Verification items for the finished model (mm, model axes). Coordinates: 2 decimals unless noted, no trailing zeros. Order: outer loops, then holes, each group sorted by start corner. A loop starts at its lowest first (then second) coordinate and runs counter-clockwise, first axis right, second up. Notation, with made-up numbers: M 59.5,38 L 83.5,38 A6 cw 83.5,47 Z; hole C 14.25,14 d2. An arc over 180 degrees is marked long. Return JSON: item names as keys, results as strings. Group by question number.
1. Section check A-A, the plane z = -25. Record the cut outline in (x, y), plus the area to 3 significant figures.
2. Section check D-D, the plane x = -93. Record the cut outline in (y, z), plus the area to 3 significant figures.
3. Material ranges on line 1 along X through (y, z) = (0.95, -31.5); line 2 along X through (y, z) = (1.9, -42.5); line 3 along Z through (x, y) = (11, 2.35), recorded low to high.
4. Mould release check, pull along X, two halves, no side actions. Record for faces 1 (the flat face through (103.7, 1.5, -24.9)), 2 (the flat face through (2, 3, 1)), 3 (the cylindrical face through (106.22, 1.48, -70.07)): +X half, -X half, draft (parallel to the pull), parting line (faces both ways), or undercut.
5. Gauge pin test, flat ends, axial feed: pin 1 (0.9 mm diameter, centred on x = 1, y = 1.5, fed in from +Z); pin 2 (1.5 mm diameter, centred on y = 1, z = -13, fed in from -X); pin 3 (1 mm diameter, centred on y = 0.5, z = 9.5, fed in from -X). Record the tip position at first contact, or that the pin passes through.
6. Section check C-C, the plane z = -43. Record the cut outline in (x, y).
7. Section check B-B, the plane y = 2.35. Give the number of separate pieces and of enclosed holes in the cut face, plus the area to 3 significant figures.
```python
from build123d import *

# Parameters (mm, degrees)
EXTRUDE_1_DEPTH     = 3
CUT_EXTRUDE_START   = -10
CUT_EXTRUDE_1_DEPTH = 10
SKETCH_3_R          = 1.75
CUT_EXTRUDE_2_DEPTH = 10
CUT_EXTRUDE_3_DEPTH = 10


with BuildPart() as part:
    # 草图1 → 凸台-拉伸1 (new body)
    with BuildSketch(Plane(origin=(0, 0, 0), x_dir=(1, 0, 0), z_dir=(0, 1, 0))):
        with BuildLine():
            Line((-66.78059141, 154.593992167), (66.78059141, 154.593992167))
            ThreePointArc((66.78059141, 154.593992167), (85.265515034, 148.222525736), (95.898700635, 131.814498742))
            Line((95.898700635, 131.814498742), (111.265547961, 69.844672358))
            ThreePointArc((111.265547961, 69.844672358), (112.147438737, 62.624165782), (111.265547961, 55.403659207))
            Line((111.265547961, 55.403659207), (95.898700635, -6.566167178))
            ThreePointArc((95.898700635, -6.566167178), (85.265515034, -22.974194171), (66.78059141, -29.345660602))
            Line((66.78059141, -29.345660602), (-66.78059141, -29.345660602))
            ThreePointArc((-66.78059141, -29.345660602), (-85.265515034, -22.974194171), (-95.898700635, -6.566167178))
            Line((-95.898700635, -6.566167178), (-111.265547961, 55.403659207))
            ThreePointArc((-111.265547961, 55.403659207), (-112.147438737, 62.624165782), (-111.265547961, 69.844672358))
            Line((-111.265547961, 69.844672358), (-95.898700635, 131.814498742))
            ThreePointArc((-95.898700635, 131.814498742), (-85.265515034, 148.222525736), (-66.78059141, 154.593992167))
        make_face()
    extrude(amount=EXTRUDE_1_DEPTH)

    # 草图2 → 切除-拉伸1 (cut)
    with BuildSketch(Plane(origin=(0, 3, 0), x_dir=(1, 0, 0), z_dir=(0, 1, 0)).offset(CUT_EXTRUDE_START)):
        with BuildLine():
            Line((111.265547961, 69.844672358), (95.898700635, 131.814498742))
            ThreePointArc((95.898700635, 131.814498742), (85.265515034, 148.222525736), (66.78059141, 154.593992167))
            Line((66.78059141, 154.593992167), (-66.78059141, 154.593992167))
            ThreePointArc((-66.78059141, 154.593992167), (-85.265515034, 148.222525736), (-95.898700635, 131.814498742))
            Line((-95.898700635, 131.814498742), (-111.265547961, 69.844672358))
            ThreePointArc((-111.265547961, 69.844672358), (-111.926149897, 66.261247255), (-112.147438737, 62.624165782))
            ThreePointArc((-112.147438737, 62.624165782), (-106.361047775, 70.035823246), (-97.766986015, 66.220447882))
            ThreePointArc((-97.766986015, 66.220447882), (0, 7.570427798), (97.766986015, 66.220447882))
            ThreePointArc((97.766986015, 66.220447882), (106.361047775, 70.035823246), (112.147438737, 62.624165782))
            ThreePointArc((112.147438737, 62.624165782), (111.926149897, 66.261247255), (111.265547961, 69.844672358))
        make_face()
    extrude(amount=CUT_EXTRUDE_1_DEPTH, mode=Mode.SUBTRACT)

    # 草图3 → 切除-拉伸2 (cut)
    with BuildSketch(Plane(origin=(0, 3, 0), x_dir=(1, 0, 0), z_dir=(0, 1, 0))):
        with Locations(Location((-80.450184708, -16.818951307, 0), (0, 0, 270))):
            Circle(SKETCH_3_R)
        with Locations(Location((-104.507530951, 62.624165782, 0), (0, 0, 270))):
            Circle(SKETCH_3_R)
        with Locations(Location((104.507530951, 62.624165782, 0), (0, 0, 270))):
            Circle(SKETCH_3_R)
        with Locations(Location((80.450184708, -16.818951307, 0), (0, 0, 270))):
            Circle(SKETCH_3_R)
    extrude(amount=-CUT_EXTRUDE_2_DEPTH, mode=Mode.SUBTRACT)

    # 草图4 → 切除-拉伸3 (cut)
    with BuildSketch(Plane(origin=(0, 3, 0), x_dir=(1, 0, 0), z_dir=(0, 1, 0))):
        with BuildLine():
            Line((11.016648097, -20.513898252), (-11.016648097, -20.513898252))
            ThreePointArc((-11.016648097, -20.513898252), (-13.814702514, -21.911306641), (-14.378457093, -24.987674549))
            add(Edge.make_bspline(
                [(-14.378457093, -24.987674549), (-14.050661547, -26.11933694), (-10.489346867, -26.76009099), (-7.724749574, -26.493757466), (-5.904508816, -27.417302496), (-5.804576355, -27.473305111)],
                knots=[0, 0, 0, 0, 0.274123853, 0.745489655, 0.777393608, 0.777393608, 0.777393608, 0.777393608], degree=3))
            ThreePointArc((-5.804576355, -27.473305111), (-5.325885634, -28.59829127), (-6.293448421, -29.345660602))
            Line((-6.293448421, -29.345660602), (6.293448421, -29.345660602))
            ThreePointArc((6.293448421, -29.345660602), (5.325885634, -28.59829127), (5.804576355, -27.473305111))
            add(Edge.make_bspline(
                [(5.804576355, -27.473305111), (5.904508816, -27.417302496), (7.724749574, -26.493757466), (10.489346867, -26.76009099), (14.050661547, -26.11933694), (14.378457093, -24.987674549)],
                knots=[0, 0, 0, 0, 0.031903952, 0.503269754, 0.777393608, 0.777393608, 0.777393608, 0.777393608], degree=3))
            ThreePointArc((14.378457093, -24.987674549), (13.814702514, -21.911306641), (11.016648097, -20.513898252))
        make_face()
    extrude(amount=-CUT_EXTRUDE_3_DEPTH, mode=Mode.SUBTRACT)


solid = part.part
```
Answers follow:
{
 "1": {"outline": "M -103.73,0 L -59.66,0 L -59.66,3 L -103.73,3 Z; M 59.66,0 L 103.73,0 L 103.73,3 L 59.66,3 Z", "area": "264 mm^2"},
 "2": {"outline": "M 0,-58.13 L 3,-58.13 L 3,13.92 L 0,13.92 Z", "area": "216 mm^2"},
 "3": {"line 1": "-105.34 to -68.78, 68.78 to 105.34", "line 2": "-108.07 to -80.75, 80.75 to 108.07", "line 3": "-8.12 to 20.51, 26.52 to 29.35"},
 "4": {"face 1": "+X half", "face 2": "draft", "face 3": "undercut"},
 "5": {"pin 1": "z = 20.51", "pin 2": "x = -100.94", "pin 3": "x = -95.18"},
 "6": {"outline": "M -108.19,0 L -81.22,0 L -81.22,3 L -108.19,3 Z; M 81.22,0 L 108.19,0 L 108.19,3 L 81.22,3 Z"},
 "7": {"separate pieces": "1", "enclosed holes": "4", "area": "11,000 mm^2"}
}
